Can you work these out from the model? Positions are in its coordinate system, mm. Face numbers are marked on the shaded views. A direction names the side the tool comes from. Coordinates: 2 decimals unless noted, no trailing zeros. Loops run counter-clockwise (first coordinate to the right, second up) from the corner with the lowest first, then second, coordinate; pieces in that order, holes last. Notation, with made-up numbers: (43, -33.75) - (60, -33.75) arc R22 cw to (60, -3.75) - close; hole circle Ø9 at (18, 4.25). An arc over 180 degrees is marked (long way). Put each result on its own line as item: value. Start each with the question number.
Solid Edge part; units mm, degrees
sketch "Sketch1" plane through (0, 0, 0) normal (0, -1, 0) x (1, 0, 0)
  line L0 (2.5, 0) -> (2.5, 15)
  line L1 (2.5, 15) -> (0, 15)
  line L2 (0, 15) -> (0, 0)
  line L3 (0, 0) -> (2.5, 0)
extrude "Protrusion1" add sketch "Sketch1" against normal blind 35
sketch "Sketch2" plane through (1.25, 0, 7.5) normal (0, -1, 0) x (0, 0, 1)
  line L0 (6.5, -1.25) -> (6.5, 0)
  line L1 (6.5, 0) -> (5.5, 0)
  line L2 (5.5, 0) -> (5.5, -1.25)
  line L3 (6.5, -1.25) -> (5.5, -1.25)
extrude "Vyříznutí_1" cut sketch "Sketch2" against normal blind 35
sketch "Sketch3" plane through (1.25, 0, 7.5) normal (0, -1, 0) x (0, 0, -1)
  line L0 (7.5, -0.25) -> (7.5, 0.5)
  line L1 (10, 0.5) -> (7.5, 0.5)
  line L2 (10, 1.25) -> (10, 0.5)
  line L3 (10.5, 1.25) -> (10, 1.25)
  line L4 (10.5, -0.25) -> (10.5, 1.25)
  line L5 (7.5, -0.25) -> (10.5, -0.25)
extrude "Vysunutí_2" add sketch "Sketch3" against normal blind 35
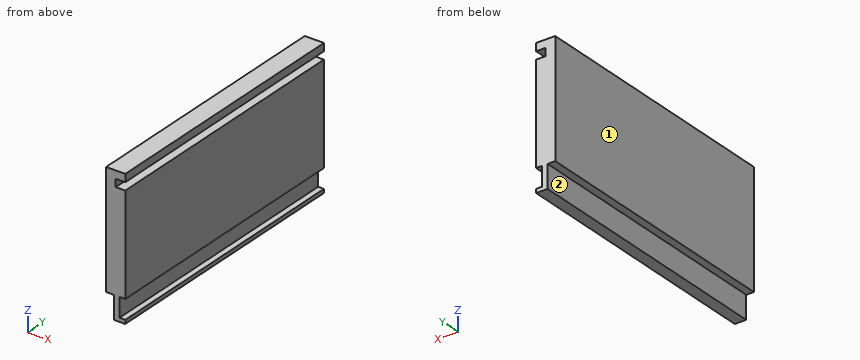
Q1. I want a section at A-A on y = 23.5. List the corners of the cut face in (x, z) for me.
Q2. I want a section at C-C on x = 0.6. List the corners of the cut face in (y, z) for me, and give its area (3 significant figures).
Q3. Please list where these lines run through material, in increasing order: line 1 along Z through (x, y) = (1.35, 17); line 2 along Z through (x, y) = (2.35, 12.5); line 3 along X through (y, z) = (7, -0.5). Write a range as [from, to].
Q4. I want a section at B-B on z = 13.5. List the corners of the cut face in (x, y) for me, and give its area (4 significant figures).
Q5. On a 3-axis mill with a long thin cutter (end or side, diameter ignored), from which of +Z, -Z, +X, -X, +Y, -Y can I reach the whole of each face in a straight line? I mean the marked faces 1 and 2. Say none if no direction works.
Q6. Will these pins go through, and if not, where does the flat tip stop? pin 1 (8 mm diameter, centred on y = 9.5, z = 1, fed in from -X); pin 2 (0.8 mm diameter, centred on y = 11, z = -1.5, fed in from +X); pin 3 (0.9 mm diameter, centred on y = 24.5, z = -1.5, fed in from -X); pin 4 (0.5 mm diameter, centred on x = 0.5, y = 21.5, fed in from -Z).
Calculated:
1. outline: (0, 0) - (1, 0) - (1, -3) - (2.5, -3) - (2.5, -2.5) - (1.75, -2.5) - (1.75, 0) - (2.5, 0) - (2.5, 13) - (1.25, 13) - (1.25, 14) - (2.5, 14) - (2.5, 15) - (0, 15) - close
2. outline: (0, 0) - (35, 0) - (35, 15) - (0, 15) - close
2. area: 525 mm2
3. line 1: [-3, 13], [14, 15]
3. line 2: [-3, -2.5], [0, 13], [14, 15]
3. line 3: [1, 1.75]
4. outline: (0, 0) - (1.25, 0) - (1.25, 35) - (0, 35) - close
4. area: 43.75 mm2
5. face 1: +Z, -Z, -X, +Y, -Y
5. face 2: -Z, -X, +Y, -Y
6. pin 1: x = 0
6. pin 2: x = 1.75
6. pin 3: x = 1
6. pin 4: z = 0
